Geometry check sheet. Reference: the model listing, model coordinates, mm. A direction names the side the tool comes from. Round coordinates to 2 decimals unless told otherwise and drop trailing zeros. Write each loop counter-clockwise with the first axis right and the second up, starting at its lowest first coordinate (ties: lowest second). Pieces come first, ordered by that corner, then holes. Notation, with made-up numbers: (74, -33) - (88, -33) arc R29 cw to (88, -12) - close; hole circle Ø7 at (-24.75, 61.25). An arc over 180 degrees is marked (long way). Return JSON: item names as keys, results as strings. Group by question number.
from build123d import *

# Parameters (mm, degrees)
BOX_W                                = 145
BOX_H                                = 182
BOX_DEPTH                            = 4
BOX001_W                             = 98
BOX001_H                             = 164
BOX001_DEPTH                         = 5
CYLINDER_R                           = 6
CYLINDER_DEPTH                       = 12
CYLINDER001_R                        = 1.75
CYLINDER001_DEPTH                    = 12
LINEARPATTERN_COUNT                  = 8
LINEARPATTERN_PITCH                  = 20
CYLINDER003_R                        = 1
CYLINDER003_DEPTH                    = 6
CYLINDER003_LINEARPATTERN004_2_R     = 1
CYLINDER003_LINEARPATTERN004_2_DEPTH = 6
LINEARPATTERN005_COUNT               = 2
LINEARPATTERN005_PITCH               = 170


with BuildPart() as part:
    # Box → Box (join)
    with BuildSketch(Plane.XY):
        with Locations((72.5, 91)):
            Rectangle(BOX_W, BOX_H)
    extrude(amount=BOX_DEPTH)

    # Box001 → Box001 (cut)
    with BuildSketch(Plane(origin=(25.5, 6, -1), x_dir=(1, 0, 0), z_dir=(0, 0, 1))):
        with Locations((49, 82)):
            Rectangle(BOX001_W, BOX001_H)
    extrude(amount=BOX001_DEPTH, mode=Mode.SUBTRACT)

    # Cylinder → Cylinder (cut)
    with BuildSketch(Plane(origin=(9, 20, -7), x_dir=(1, 0, 0), z_dir=(0, 0, 1))):
        Circle(CYLINDER_R)
    cylinder = extrude(amount=CYLINDER_DEPTH, mode=Mode.SUBTRACT)

    # Cylinder001 → Cylinder001 (cut)
    with BuildSketch(Plane(origin=(18, 20, -7), x_dir=(1, 0, 0), z_dir=(0, 0, 1))):
        Circle(CYLINDER001_R)
    cylinder001 = extrude(amount=CYLINDER001_DEPTH, mode=Mode.SUBTRACT)

    # LinearPattern: Cylinder, Cylinder001 ×8
    with Locations(*[(0, i * LINEARPATTERN_PITCH, 0) for i in range(1, LINEARPATTERN_COUNT)]):
        add(cylinder, mode=Mode.SUBTRACT)
        add(cylinder001, mode=Mode.SUBTRACT)

    # Cylinder003 → Cylinder003 (cut)
    with BuildSketch(Plane(origin=(5, 5, -3), x_dir=(1, 0, 0), z_dir=(0, 0, 1))):
        Circle(CYLINDER003_R)
    cylinder003 = extrude(amount=CYLINDER003_DEPTH, mode=Mode.SUBTRACT)

    # Cylinder003 LinearPattern004 2 → Cylinder003 LinearPattern004 2 (cut)
    with BuildSketch(Plane(origin=(138, 5, -3), x_dir=(1, 0, 0), z_dir=(0, 0, 1))):
        Circle(CYLINDER003_LINEARPATTERN004_2_R)
    cylinder003_linearpattern004_2 = extrude(amount=CYLINDER003_LINEARPATTERN004_2_DEPTH, mode=Mode.SUBTRACT)

    # LinearPattern005: Cylinder003, Cylinder003 LinearPattern004 2 ×2
    with Locations(*[(0, i * LINEARPATTERN005_PITCH, 0) for i in range(1, LINEARPATTERN005_COUNT)]):
        add(cylinder003, mode=Mode.SUBTRACT)
        add(cylinder003_linearpattern004_2, mode=Mode.SUBTRACT)


with BuildPart() as part_1:
    # Body placement: moved
    add(part.part.moved(Location((0, 0, 4))))


solid = part_1.part
1. Depth check by flat-ended pin: pin 1 Ø11 at (x, y) = (9, 20) entering from -Z (1 decimal). Enter the tip coordinate at first touch or a pass-through.
2. Section check C-C (z = 4.7). State how many separate pieces and enclosed holes the cut face has, and give its area (3 significant figures).
3. Material ranges on line 1 along X through (y, z) = (20, 7.05); line 2 along Y through (x, z) = (106, 7.45); line 3 along X through (y, z) = (30, 6.9), recorded low to high.
4. Mould release check, pull along Y, two halves, no side actions. Record for faces 1 (the face through (123.5, 87, 6)), 2 (the face through (23, 112, 8)), 3 (the face through (71, 182, 6)): pulls with the +Y half, pulls with the -Y half, needs draft (parallel to the pull), parting line crosses it, or undercut.
5. Section check B-B (y = 30). Enter the section's corners in (x, z), and give its area (3 significant figures).
6. Section check A-A (x = 62). Enter the section's corners in (y, z), and give its area (3 significant figures).
7. Tool access check on faces 4 (the face through (74, 6, 6)), 5 (the face through (71, 0, 6)). Record the directions out of +Z, -Z, +X, -X, +Y, -Y that give a thin tool (end or side, any length) a straight path to the whole face; none if there is none.
Result sheet:
{
 "1": {"pin 1": "passes through"},
 "2": {"separate pieces": "1", "enclosed holes": "21", "area": "9,320 mm²"},
 "3": {"line 1": "x = 0 to 3, 15 to 16.25, 19.75 to 25.5, 123.5 to 145", "line 2": "y = 0 to 6, 170 to 182", "line 3": "x = 0 to 25.5, 123.5 to 145"},
 "4": {"face 1": "undercut", "face 2": "needs draft", "face 3": "pulls with the +Y half"},
 "5": {"outline": "(0, 4) - (25.5, 4) - (25.5, 8) - (0, 8) - close; (123.5, 4) - (145, 4) - (145, 8) - (123.5, 8) - close", "area": "188 mm²"},
 "6": {"outline": "(0, 4) - (6, 4) - (6, 8) - (0, 8) - close; (170, 4) - (182, 4) - (182, 8) - (170, 8) - close", "area": "72.0 mm²"},
 "7": {"face 4": "+Z, -Z", "face 5": "+Z, -Z, +X, -X, -Y"}
}
